from build123d import *

# Parameters (mm, degrees)
F1_DEPTH = 10
F2_R     = 2.65
F3_DEPTH = 30.001
F4_DEPTH = 30.001
F5_R     = 2
F6_R     = 2


with BuildPart() as f1:
    # F0 (on Top) → F1 (new body)
    with BuildSketch(Plane.XY):
        with BuildLine():
            Line((-10, 30), (-10, 19))
            ThreePointArc((-10, 19), (-14.497695, 9.397234), (-24.754098, 6.704918))
            Line((-24.754098, 6.704918), (-30.655738, 7.786885))
            ThreePointArc((-30.655738, 7.786885), (-40.943872, 13.796773), (-45, 25))
            Line((-45, 25), (-45, 30))
            Line((-45, 30), (-55, 30))
            Line((-55, 30), (-55, 0))
            Line((-55, 0), (0, 0))
            Line((0, 0), (0, 30))
            Line((0, 30), (-10, 30))
        make_face()
    extrude(amount=F1_DEPTH)

    # F2 (on face) → F3 (cut, through all)
    with BuildSketch(Plane(origin=(0, 30, 0), x_dir=(-1, 0, 0), z_dir=(0, 1, 0))):
        with Locations((50, 5)):
            Circle(F2_R)
    extrude(amount=-F3_DEPTH, mode=Mode.SUBTRACT)

    # F2 (on face) → F4 (cut, through all)
    with BuildSketch(Plane(origin=(0, 30, 0), x_dir=(-1, 0, 0), z_dir=(0, 1, 0))):
        with Locations((5, 5)):
            Circle(F2_R)
    extrude(amount=-F4_DEPTH, mode=Mode.SUBTRACT)

    # F5
    f5_edges = [f1.edges().sort_by_distance(p)[0] for p in [
        (-55, 15, 10),
        (0, 15, 10),
        (0, 15, 0),
        (-55, 15, 0),
        (-40.943872, 13.796773, 0),
        (-14.497695, 9.397234, 10),
    ]]
    fillet(f5_edges, radius=F5_R)

    # F6
    f6_edges = [f1.edges().sort_by_distance(p)[0] for p in [
        (-10, 30, 5),
        (-55, 30, 5),
    ]]
    fillet(f6_edges, radius=F6_R)


solid = f1.part
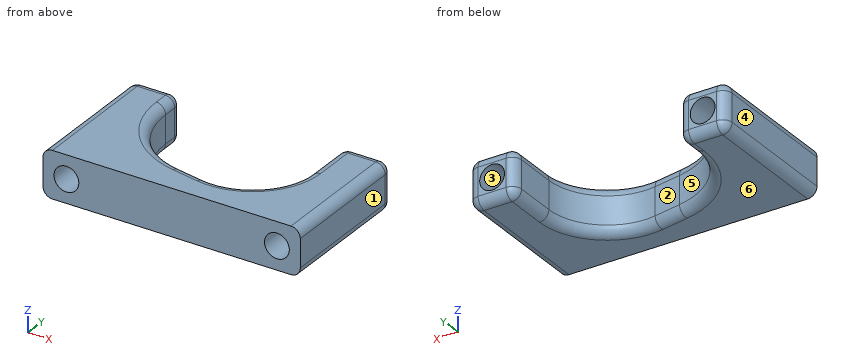
Can you work these out from the model? Positions are in its coordinate system, mm. Face numbers are marked on the shaded views. A direction names the side the tool comes from. Round coordinates to 2 decimals unless told otherwise and drop trailing zeros. Write each loop counter-clockwise with the first axis right and the second up, starting at its lowest first coordinate (ties: lowest second). Pieces come first, ordered by that corner, then holes. Notation, with made-up numbers: (13.25, 41) -> (42.25, 41) arc R31 ccw to (42.25, 73) -> close; hole circle Ø4 at (13.5, 87). An arc over 180 degrees is marked (long way). Use one line per item in the form item = value. Start each with the question number.
Q1. I'm going to push a flat-ended pin straight in: P1, Ø6, axis at x = -18.5, z = 6.5, coming from the +Y side. Where does the tip first touch, or does it pass through?
Q2. Imagine slicing it at C-C (y = 3.75). Please give me the cut outline in (x, z), then the cut area to 3 significant figures.
Q3. We'd pull the mould along X, two halves only. Please class the marked faces 3, 4, 5 and 6: +X half, -X half, draft (parallel to the pull), parting line (faces both ways), or undercut.
Q4. If I drill on probe 1 along Z at (x, y) = (-5, 16.75); probe 2 along X at (y, z) = (4.75, 6); probe 3 along X at (y, z) = (14.5, 8.5), over which ranges is the centre line in solid material (lowest first)? Write a range as [from, to].
Q5. Imagine slicing it at D-D (y = 10.75). Count the separate pieces of the cut face and the enclosed holes in it, then the cut area to 3 significant figures.
Q6. Which directions (+Z, -Z, +X, -X, +Y, -Y) give clear straight access to the entire face, cutting with the end or side of a thin tool? Please do the marked faces 1 and 2.
Q7. Imagine slicing it at B-B (x = -50). Please give me the cut outline in (y, z).
Q8. Imagine slicing it at A-A (z = 5). Please give me the cut outline in (x, y).
Worked out:
q1.P1 = 8.64
q2.outline = (-55, 2) arc R2 ccw to (-53, 0) -> (-2, 0) arc R2 ccw to (0, 2) -> (0, 8) arc R2 ccw to (-2, 10) -> (-53, 10) arc R2 ccw to (-55, 8) -> close; hole circle Ø5.3 at (-50, 5); hole circle Ø5.3 at (-5, 5)
q2.area = 502 mm^2
q3.face_3 = undercut
q3.face_4 = -X half
q3.face_5 = undercut
q3.face_6 = draft
q4.probe_1 = [0, 2.35], [7.65, 10]
q4.probe_2 = [-55, -52.45], [-47.55, -7.45], [-2.55, 0]
q4.probe_3 = [-54.94, -41.58], [-10.77, -0.06]
q5.separate_pieces = 2
q5.enclosed_holes = 2
q5.area = 252 mm^2
q6.face_1 = +Z, -Z, +X, +Y, -Y
q6.face_2 = +Z, -Z, +Y
q7.outline = (0, 0) -> (28, 0) arc R2 ccw to (30, 2) -> (30, 2.35) -> (0, 2.35) -> close; (0, 7.65) -> (30, 7.65) -> (30, 8) arc R2 ccw to (28, 10) -> (0, 10) -> close
q8.outline = (-55, 0) -> (-52.65, 0) -> (-52.65, 30) -> (-53, 30) arc R2 ccw to (-55, 28) -> close; (-47.35, 0) -> (-7.65, 0) -> (-7.65, 30) -> (-8, 30) arc R2 ccw to (-10, 28) -> (-10, 19) arc R12.5 cw to (-24.75, 6.7) -> (-30.66, 7.79) arc R17.5 cw to (-45, 25) -> (-45, 28) arc R2 ccw to (-47, 30) -> (-47.35, 30) -> close; (-2.35, 0) -> (0, 0) -> (0, 28) arc R2 ccw to (-2, 30) -> (-2.35, 30) -> close
